Verification items for the finished model (mm, model axes). A direction names the side the tool comes from. Give positions to 0.01 mm unless a question says otherwise; leave off trailing zeros. Order: outer loops, then holes, each group sorted by start corner. A loop starts at its lowest first (then second) coordinate and runs counter-clockwise, first axis right, second up. Notation, with made-up numbers: (-19, -5.5) -> (-5, -5.5) arc R10 cw to (-5, 11.5) -> close; hole circle Ø2 at (38.25, 30.25). An arc over 180 degrees is marked (long way). Return JSON: item names as keys, results as strings. Group by question number.
(1) Cross-section at A-A on z = 4. Enter the section's corners in (x, y), then the cut area to 3 significant figures.
(2) Depth check by flat-ended pin: pin 1 Ø6.5 at (y, z) = (-75, 8.5) entering from +X; pin 2 Ø4 at (y, z) = (-75, 5.5) entering from -X; pin 3 Ø8 at (x, z) = (1024, 8.5) entering from -Y. Enter the tip coordinate at first touch or a pass-through.
(3) Tool access check on faces 1 (the face through (1845, -17.178, 9)), 2 (the face through (1430, -42, 18)), 3 (the face through (1035.447, -76, 9)), 4 (the face through (1025, -17.178, 9)), 5 (the face through (1846, -67.178, 9)). Record the directions out of +Z, -Z, +X, -X, +Y, -Y that give a thin tool (end or side, any length) a straight path to the whole face; none if there is none.
(4) Thickness scan on line 1 along X through (y, z) = (-69, 3.25); line 2 along X through (y, z) = (-74, 15.75). Record the ranges inside material, lowest first.
Autodesk Inventor part; units mm, degrees
ref_plane "YZ Plane" through (0, 0, 0) normal (1, 0, 0) x (0, 1, 0)
ref_plane "XZ Plane" through (0, 0, 0) normal (0, 1, 0) x (-1, 0, 0)
ref_plane "XY Plane" through (0, 0, 0) normal (0, 0, 1) x (1, 0, 0)
sketch "Sketch1" plane through (0, 0, 0) normal (0, 0, 1) x (1, 0, 0)
  line L0 (1035.4474, -2.1782) -> (1835.4474, -2.1782)
  line L1 (1835.4474, -82.1782) -> (1035.4474, -82.1782)
  line L2 (1035.4474, -17.1782) -> (1017.4474, -17.1782)
  line L3 (1017.4474, -17.1782) -> (1017.4474, -67.1782)
  line L4 (1017.4474, -67.1782) -> (1035.4474, -67.1782)
  line L5 (1835.4474, -17.1782) -> (1853.4474, -17.1782)
  line L6 (1853.4474, -17.1782) -> (1853.4474, -67.1782)
  line L7 (1853.4474, -67.1782) -> (1835.4474, -67.1782)
  line L8 (1835.4474, -2.1782) -> (1835.4474, -17.1782)
  line L9 (1835.4474, -67.1782) -> (1835.4474, -82.1782)
  line L10 (1035.4474, -82.1782) -> (1035.4474, -67.1782)
  line L11 (1035.4474, -17.1782) -> (1035.4474, -2.1782)
  point P0 (0, 0)
  dimension "d10" = 800
  dimension "d11" = 80
  dimension "d12" = 50
  dimension "d13" = 18
  dimension "d14" = 50
  dimension "d15" = 18
  dimension "d19" = 15
  dimension "d20" = 800
  dimension "d21" = 18
extrude "Extrusion1" add sketch "Sketch1" along normal blind 18
sketch "Sketch2" plane through (0, 0, 18) normal (0, 0, 1) x (1, 0, 0)
  line L0 (1035.4474, -17.1782) -> (1034.3161, -16.0469)
  line L1 (1035.4474, -17.1782) -> (1037.0474, -17.1782) construction
  line L2 (1035.4474, -67.1782) -> (1034.3161, -68.3096)
  line L3 (1835.4474, -17.1782) -> (1836.5788, -16.0469)
  line L4 (1835.4474, -67.1782) -> (1836.5788, -68.3096)
  circle A0 centre (1836.5788, -68.3096) radius 1.6
  circle A1 centre (1836.5788, -16.0469) radius 1.6
  circle A2 centre (1034.3161, -68.3096) radius 1.6
  circle A3 centre (1034.3161, -16.0469) radius 1.6
  point P0 (0, 0)
  dimension "d22" = 1.6
  dimension "d23" = 135
  dimension "d24" = 3.2
  dimension "d25" = 3.2
  dimension "d26" = 3.2
  dimension "d27" = 3.2
extrude "Extrusion2" cut sketch "Sketch2" against normal blind 20
properties part number "viga diagonal" material "Wood (Birch)"
Verdict:
{
 "1": {"outline": "(1017.45, -67.18) -> (1033.18, -67.18) arc R1.6 cw to (1035.45, -69.44) -> (1035.45, -82.18) -> (1835.45, -82.18) -> (1835.45, -69.44) arc R1.6 cw to (1837.71, -67.18) -> (1853.45, -67.18) -> (1853.45, -17.18) -> (1837.71, -17.18) arc R1.6 cw to (1835.45, -14.92) -> (1835.45, -2.18) -> (1035.45, -2.18) -> (1035.45, -14.92) arc R1.6 cw to (1033.18, -17.18) -> (1017.45, -17.18) -> close", "area": "65,800 mm²"},
 "2": {"pin 1": "x = 1835.45", "pin 2": "x = 1035.45", "pin 3": "y = -67.18"},
 "3": {"face 1": "+Z, -Z, +X, +Y", "face 2": "+Z, +X, -X, +Y, -Y", "face 3": "+Z, -Z, -X, -Y", "face 4": "+Z, -Z, -X, +Y", "face 5": "+Z, -Z, +X, -Y"},
 "4": {"line 1": "1035.76 to 1835.14", "line 2": "1035.45 to 1835.45"}
}
